from build123d import *

# Parameters (mm, degrees)
ESQUISSE1_R             = 3.5
BOSS_EXTRU_1_DEPTH      = 5
ESQUISSE2_R             = 3.5
ESQUISSE2_R_2           = 1.5
BOSS_EXTRU_2_DEPTH      = 5
ESQUISSE3_R             = 1.5
ENL_V_MAT_EXTRU_1_DEPTH = 52.599228309
BOSS_EXTRU_3_DEPTH      = 5


with BuildPart() as part:
    # Esquisse1 → Boss.-Extru.1 (new body)
    with BuildSketch(Plane.XY):
        with BuildLine():
            Line((-26.278959381, 12.43097678), (-23.625738837, 9.777756236))
            ThreePointArc((-23.625738837, 9.777756236), (-22.982271103, 8.820887218), (-22.747269794, 7.691983578))
            ThreePointArc((-22.747269794, 7.691983578), (-2.226699014, -26.772009928), (37.87835279, -26.104557126))
            ThreePointArc((37.87835279, -26.104557126), (39.583612673, -19.242189551), (32.721245099, -17.536929668))
            ThreePointArc((32.721245099, -17.536929668), (5.06736173, -19.249102003), (-12.195220044, 2.422816923))
            ThreePointArc((-12.195220044, 2.422816923), (-15.15644736, 10.772312527), (-20.427158676, 17.892884575))
            Line((-20.427158676, 17.892884575), (-20.622105131, 18.08783103))
            ThreePointArc((-20.622105131, 18.08783103), (-35.933936854, 27.742808503), (-26.278959381, 12.43097678))
        make_face()
        with Locations((-29.371809148, 21.180680797)):
            Circle(ESQUISSE1_R, mode=Mode.SUBTRACT)
    extrude(amount=BOSS_EXTRU_1_DEPTH)

    # Esquisse2 → Boss.-Extru.2 (add, through all)
    with BuildSketch(Plane.XY.offset(5)):
        with Locations((-29.371809148, 21.180680797)):
            Circle(ESQUISSE2_R)
        with Locations((-29.371809148, 21.180680797)):
            Circle(ESQUISSE2_R_2, mode=Mode.SUBTRACT)
    extrude(amount=-BOSS_EXTRU_2_DEPTH)

    # Esquisse3 → Enlèv. mat.-Extru.1 (cut, through all)
    with BuildSketch(Plane.XY.offset(5)):
        with Locations((35.299798944, -21.820743397)):
            Circle(ESQUISSE3_R)
        with Locations((1.420331358, -23.010555966)):
            Circle(ESQUISSE3_R)
        with Locations((-16.690323797, -0.244656241)):
            Circle(ESQUISSE3_R)
    extrude(amount=-ENL_V_MAT_EXTRU_1_DEPTH, mode=Mode.SUBTRACT)

    # Esquisse4 → Boss.-Extru.3 (add, through all)
    with BuildSketch(Plane(origin=(0, 0, 0), x_dir=(-1, 0, 0), z_dir=(0, 0, -1))):
        with BuildLine():
            ThreePointArc((-32.721245099, -17.536929668), (-31.583474438, -18.188350077), (-30.418328753, -18.789437557))
            Line((-30.418328753, -18.789437557), (-29.651415378, -17.296811968))
            ThreePointArc((-29.651415378, -17.296811968), (-29.778275742, -16.192937164), (-30.846670439, -15.887706259))
            Line((-30.846670439, -15.887706259), (-33.82002484, -16.842679657))
            Line((-33.82002484, -16.842679657), (-34.160934368, -16.952171997))
            ThreePointArc((-34.160934368, -16.952171997), (-33.418234352, -17.188280263), (-32.721245099, -17.536929668))
        make_face()
        with BuildLine():
            ThreePointArc((-30.141880226, -18.922742606), (-28.344838513, -19.707023958), (-26.500403555, -20.372242602))
            Line((-26.500403555, -20.372242602), (-25.950815291, -18.786670146))
            ThreePointArc((-25.950815291, -18.786670146), (-26.231514379, -17.711569612), (-27.332196648, -17.559478592))
            Line((-27.332196648, -17.559478592), (-30.141880226, -18.922742606))
        make_face()
        with BuildLine():
            ThreePointArc((-26.207967618, -20.465383608), (-24.318558502, -20.989396346), (-22.398954871, -21.388868572))
            Line((-22.398954871, -21.388868572), (-22.07759519, -19.741805965))
            ThreePointArc((-22.07759519, -19.741805965), (-22.506564116, -18.716808992), (-23.617697141, -18.720875242))
            Line((-23.617697141, -18.720875242), (-26.207967618, -20.465383608))
        make_face()
        with BuildLine():
            ThreePointArc((-22.096333261, -21.439997678), (-20.152041379, -21.693345733), (-18.195352752, -21.819146273))
            Line((-18.195352752, -21.819146273), (-18.108597219, -20.143270158))
            ThreePointArc((-18.108597219, -20.143270158), (-18.677325521, -19.188712012), (-19.776865153, -19.348854862))
            Line((-19.776865153, -19.348854862), (-22.096333261, -21.439997678))
        make_face()
        with BuildLine():
            ThreePointArc((-17.888549284, -21.827249111), (-15.927948113, -21.804906224), (-13.972993908, -21.654539278))
            Line((-13.972993908, -21.654539278), (-14.122563696, -19.983097938))
            ThreePointArc((-14.122563696, -19.983097938), (-14.819768177, -19.117916427), (-15.88590027, -19.430958747))
            Line((-15.88590027, -19.430958747), (-17.888549284, -21.827249111))
        make_face()
        with BuildLine():
            ThreePointArc((-13.668095361, -21.619455093), (-11.730081941, -21.321864532), (-9.815647169, -20.898313282))
            Line((-9.815647169, -20.898313282), (-10.19857491, -19.264467016))
            ThreePointArc((-10.19857491, -19.264467016), (-11.010423491, -18.505826774), (-12.021996685, -18.96555801))
            Line((-12.021996685, -18.96555801), (-13.668095361, -21.619455093))
        make_face()
        with BuildLine():
            ThreePointArc((-9.51870253, -20.820738122), (-7.641725776, -20.253803889), (-5.805791566, -19.565471313))
            Line((-5.805791566, -19.565471313), (-6.414480226, -18.00163456))
            ThreePointArc((-6.414480226, -18.00163456), (-7.324866364, -17.364586511), (-8.261811709, -17.961885897))
            Line((-8.261811709, -17.961885897), (-9.51870253, -20.820738122))
        make_face()
        with BuildLine():
            ThreePointArc((-5.522692022, -19.446944218), (-3.743989923, -18.621913915), (-2.022980005, -17.68245608))
            Line((-2.022980005, -17.68245608), (-2.8453536, -16.219654336))
            ThreePointArc((-2.8453536, -16.219654336), (-3.836215831, -15.716837097), (-4.679944946, -16.439854603))
            Line((-4.679944946, -16.439854603), (-5.522692022, -19.446944218))
        make_face()
        with BuildLine():
            ThreePointArc((-1.759342065, -17.52532855), (-0.114202903, -16.458570238), (1.457739014, -15.286625373))
            Line((1.457739014, -15.286625373), (0.437995836, -13.953879663))
            ThreePointArc((0.437995836, -13.953879663), (-0.61368443, -13.595268797), (-1.347458283, -14.429660233))
            Line((-1.347458283, -14.429660233), (-1.759342065, -17.52532855))
        make_face()
        with BuildLine():
            Line((9.503225829, 1.258047301), (11.195220044, -1.366827201))
            ThreePointArc((11.195220044, -1.366827201), (11.75717366, 0.511646725), (12.195220044, 2.422816923))
            Line((12.195220044, 2.422816923), (10.554962651, 2.777278429))
            ThreePointArc((10.554962651, 2.777278429), (9.521535347, 2.369036904), (9.503225829, 1.258047301))
        make_face()
        with BuildLine():
            ThreePointArc((9.573674437, -5.268877882), (10.393983884, -3.487993672), (11.096209126, -1.657328255))
            Line((11.096209126, -1.657328255), (9.522025266, -1.075922675))
            ThreePointArc((9.522025266, -1.075922675), (8.44149028, -1.334915489), (8.267265601, -2.432311906))
            Line((8.267265601, -2.432311906), (9.573674437, -5.268877882))
        make_face()
        with BuildLine():
            ThreePointArc((7.419966271, -8.904390336), (8.482357148, -7.256427417), (9.43482956, -5.542585982))
            Line((9.43482956, -5.542585982), (7.957950007, -4.745771034))
            ThreePointArc((7.957950007, -4.745771034), (6.851744443, -4.850376889), (6.525061109, -5.912408496))
            Line((6.525061109, -5.912408496), (7.419966271, -8.904390336))
        make_face()
        with BuildLine():
            ThreePointArc((4.776823702, -12.201238381), (6.060218871, -10.718891256), (7.244042024, -9.155875293))
            Line((7.244042024, -9.155875293), (5.893767102, -8.159459262))
            ThreePointArc((5.893767102, -8.159459262), (4.783837353, -8.107602847), (4.311176546, -9.113199633))
            Line((4.311176546, -9.113199633), (4.776823702, -12.201238381))
        make_face()
        with BuildLine():
            ThreePointArc((1.696684946, -15.094014714), (3.175622689, -13.806692179), (4.567310309, -12.425510899))
            Line((4.567310309, -12.425510899), (3.370428584, -11.249262026))
            ThreePointArc((3.370428584, -11.249262026), (2.278794929, -11.041972137), (1.66953393, -11.971183722))
            Line((1.66953393, -11.971183722), (1.696684946, -15.094014714))
        make_face()
    extrude(amount=-BOSS_EXTRU_3_DEPTH)


solid = part.part
Could you check a few things on this model? Use its own coordinates, in mm. A direction names the side the tool comes from. Give positions to 0.01 mm unless a question says otherwise; leave off trailing zeros. Order: outer loops, then holes, each group sorted by start corner. A loop starts at its lowest first (then second) coordinate and runs counter-clockwise, first axis right, second up. Notation, with made-up numbers: (-16, 58.25) - (-12, 58.25) arc R14 ccw to (-12, 78.25) - close; hole circle Ø7 at (48, 64). An arc over 180 degrees is marked (long way). Return JSON: item names as keys, results as strings. Group by question number.
Q1. Suppose I cut it at D-D, the plane x = 15. Please give me the cut outline in (y, z).
Q2. Suppose I cut it at B-B, the plane z = 3.8. State how many separate pieces and enclosed holes the cut face has, and give its area (3 significant figures).
Q3. Please list where these lines run through material, in increasing order: line 1 along X through (y, z) = (22.5, 4.5); line 2 along Y through (x, z) = (20.5, 3.1); line 3 along Y through (x, z) = (-25, 1.7). Write a range as [from, to].
Q4. Thinking about a two-plate mould opening in Y: for faces 3 (the face through (22.24, -20.58, 2.46)), 4 (the face through (10.004, -20.093, 2.465)), 5 (the face through (28.717, -18.232, 2.465)), 6 (the face through (-24.97, 11.12, 2.46)), which applies, pulls with the +Y half, pulls with the -Y half, needs draft (parallel to the pull), parting line crosses it, or undercut?
Q5. Which directions (+Z, -Z, +X, -X, +Y, -Y) give clear straight access to the entire face, cutting with the end or side of a thin tool? Please do faces 1 (the face through (-8.91, -3.83, 2.46)), 2 (the face through (12.83, -20.27, 2.46)).
Q6. Suppose I cut it at A-A, the plane x = -29. Please give me the cut outline in (y, z), and give its area (3 significant figures).
Q7. Will these pins go through, and if not, where does the flat tip stop? pin 1 Ø2.5 at (x, y) = (-29.37, 21.18) entering from -Z; pin 2 Ø1 at (x, z) = (29, 2.5) entering from -Y.
Q8. Suppose I cut it at C-C, the plane y = 24. Please give me the cut outline in (x, z).
Resolved:
{
 "1": {"outline": "(-31.77, 0) - (-19.08, 0) - (-19.08, 5) - (-31.77, 5) - close"},
 "2": {"separate pieces": "1", "enclosed holes": "4", "area": "1,180 mm2"},
 "3": {"line 1": "x = [-38.56, -30.09], [-28.66, -20.19]", "line 2": "y = [-31.7, -20]", "line 3": "y = [11.15, 29.37]"},
 "4": {"face 3": "undercut", "face 4": "pulls with the +Y half", "face 5": "undercut", "face 6": "pulls with the -Y half"},
 "5": {"face 1": "+Z, -Z", "face 2": "+Z, -Z, +Y"},
 "6": {"outline": "(11.91, 0) - (19.73, 0) - (19.73, 5) - (11.91, 5) - close; (22.63, 0) - (30.45, 0) - (30.45, 5) - (22.63, 5) - close", "area": "78.2 mm2"},
 "7": {"pin 1": "passes through", "pin 2": "stops at y = -30.22"},
 "8": {"outline": "(-38.21, 0) - (-20.53, 0) - (-20.53, 5) - (-38.21, 5) - close"}
}
